from build123d import *

# Parameters (mm, degrees)
BOSS_EXTRUDE1_DEPTH      = 38
BOSS_EXTRUDE2_DEPTH      = 14
BOSS_EXTRUDE5_DEPTH      = 10
BOSS_EXTRUDE5_DEPTH_BACK = 38
SKETCH6_R                = 2
CUT_EXTRUDE2_DEPTH       = 36


with BuildPart() as part:
    # Sketch1 → Boss-Extrude1 (new body)
    with BuildSketch(Plane.XY):
        with BuildLine():
            Line((22.631743337, -14.12565234), (22.631743337, 13.87434766))
            Line((22.631743337, 13.87434766), (1.698298535, 18.39987252))
            ThreePointArc((1.698298535, 18.39987252), (-0.292783652, 18.720543399), (-2.306666921, 18.827838622))
            ThreePointArc((-2.306666921, 18.827838622), (-21.260157884, -0.12565234), (-2.306666921, -19.079143303))
            ThreePointArc((-2.306666921, -19.079143303), (-0.292783652, -18.971848079), (1.698298535, -18.651177201))
            Line((1.698298535, -18.651177201), (22.631743337, -14.12565234))
        make_face()
        with BuildLine():
            Line((17.644061285, -10.101016443), (17.644061285, 9.849711763))
            Line((17.644061285, 9.849711763), (0.644376893, 13.52481135))
            ThreePointArc((0.644376893, 13.52481135), (-0.822744568, 13.761096487), (-2.306666921, 13.840156571))
            ThreePointArc((-2.306666921, 13.840156571), (-16.272475832, -0.12565234), (-2.306666921, -14.091461251))
            ThreePointArc((-2.306666921, -14.091461251), (-0.822744568, -14.012401167), (0.644376893, -13.77611603))
            Line((0.644376893, -13.77611603), (17.644061285, -10.101016443))
        make_face(mode=Mode.SUBTRACT)
    extrude(amount=BOSS_EXTRUDE1_DEPTH)

    # Sketch2 → Boss-Extrude2 (add, symmetric)
    with BuildSketch(Plane(origin=(0, 0, 0), x_dir=(1, 0, 0), z_dir=(0, 1, 0))):
        Polygon((22.631743337, -38), (22.631743337, 0), (48.276983868, 0), (42.631743337, -38), align=None)
    extrude(amount=BOSS_EXTRUDE2_DEPTH, both=True)

    # Sketch4 → Boss-Extrude5 (add, two sides: drawn at the far end of the back side and taken through both)
    with BuildSketch(Plane(origin=(0, 14, 0), x_dir=(1, 0, 0), z_dir=(0, 1, 0)).offset(-BOSS_EXTRUDE5_DEPTH_BACK)):
        Polygon((28.899463429, 0), (22.957104975, -40), (48.666190602, -40), (54.608549056, 0), align=None)
    extrude(amount=BOSS_EXTRUDE5_DEPTH + BOSS_EXTRUDE5_DEPTH_BACK)

    # Sketch6 → Cut-Extrude2 (cut)
    with BuildSketch(Plane(origin=(28.275431305, 0, 4.200568706), x_dir=(-0.14694627579900546, 0, 0.9891444748007253), z_dir=(-0.9891444748007252, 0, -0.14694627579900543))):
        with Locations((0.974565013, 19)):
            Circle(SKETCH6_R)
        with Locations((29.583142195, 19)):
            Circle(SKETCH6_R)
        with Locations((0.974565013, -19)):
            Circle(SKETCH6_R)
        with Locations((29.583142195, -19)):
            Circle(SKETCH6_R)
    extrude(amount=-CUT_EXTRUDE2_DEPTH, mode=Mode.SUBTRACT)


solid = part.part
Read the model definition and answer for the solid it produces. Units are mm, in the model's axes. A direction names the side the tool comes from. Give positions to 0.01 mm unless a question says otherwise; leave off trailing zeros. Write each loop counter-clockwise with the first axis right and the second up, starting at its lowest first coordinate (ties: lowest second). Pieces come first, ordered by that corner, then holes. Notation, with made-up numbers: M 62,2.25 L 73,2.25 A31 cw 73,32.25 Z; hole C 88.5,88 d10. An arc over 180 degrees is marked long. One line per item, written item: value. Start each with the question number.
(1) Find the intervals of material crossed by line 1 (Z direction, x = -14, y = -15); line 2 (X direction, y = -2.5, z = 31.5); line 3 (Y direction, x = -5.5, z = 36), in increasing order.
(2) Find section C-C (z = 26.5). Determine the outline of the cut face in (x, y), plus the area to 3 significant figures.
(3) Find section D-D (y = -12). Determine the outline of the cut face in (x, z).
(4) Find section A-A (y = 16). Determine the outline of the cut face in (x, z).
(5) Determine the mould class of faces 1 (the cylindrical face through (36.367, 20.983, 35.047)), 2 (the flat face through (9.025, -11.964, 18.734)), 3 (the flat face through (25, 14, 15)), 4 (the flat face through (36, 0, 40)) for opening direction Y: pulls with the +Y half, pulls with the -Y half, needs draft (parallel to the pull), parting line crosses it, or undercut.
(6) A tool of negligible diameter and unlimited length cuts with its end or side. For faces 5 (the flat face through (25, -14, 15)), 6 (the flat face through (12.312, 16.105, 18.734)), 7 (the flat face through (12.02, -16.42, 18.73)), 8 (the flat face through (17.644, 0, 19)), from which of +Z, -Z, +X, -X, +Y, -Y can it reach the whole face along a straight path? Write none if from no direction.
(7) Flat-ended cylindrical pins translate along their axes: pin 1 Ø19 at (x, y) = (-4.5, 0.5) entering from +Z; pin 2 Ø4 at (x, y) = (6, 11) entering from +Z; pin 3 Ø3 at (y, z) = (-13.5, 16.5) entering from -X; pin 4 Ø1.5 at (y, z) = (14.5, 34) entering from +X. Find the tip coordinate at first contact, or state that the pin passes through.
(8) Find section B-B (x = -11.5). Determine the outline of the cut face in (y, z), plus the area to 3 significant figures.
Results below:
1. line 1: z = 0 to 38
1. line 2: x = -21.11 to -16.07, 17.64 to 49.93
1. line 3: y = -18.81 to -13.72, 13.47 to 18.56
2. outline: M 1.7,-18.65 L 22.63,-14.13 L 22.63,-14 L 24.96,-14 L 24.96,-24 L 50.67,-24 L 50.67,24 L 24.96,24 L 24.96,14 L 22.63,14 L 22.63,13.87 L 1.7,18.4 A18.95 ccw long Z; hole M 0.64,-13.78 L 17.64,-10.1 L 17.64,9.85 L 0.64,13.52 A13.97 ccw long Z
2. area: 1,910 mm^2
3. outline: M -17.08,0 L -9.66,0 L -9.66,38 L -17.08,38 Z; M 8.86,0 L 54.61,0 L 48.67,40 L 22.96,40 L 23.25,38 L 8.86,38 Z
4. outline: M -12.27,0 L 12.8,0 L 12.8,38 L -12.27,38 Z; M 22.96,40 L 28.9,0 L 54.61,0 L 48.67,40 Z
5. face 1: undercut
5. face 2: undercut
5. face 3: pulls with the +Y half
5. face 4: needs draft
6. face 5: -Z, -Y
6. face 6: +Z, -Z, +Y
6. face 7: +Z, -Z, -Y
6. face 8: +Z, -Z
7. pin 1: passes through
7. pin 2: stops at z = 38
7. pin 3: stops at x = -17.08
7. pin 4: stops at x = 49.67
8. outline: M -16.7,0 L -10.64,0 L -10.64,38 L -16.7,38 Z; M 10.39,0 L 16.45,0 L 16.45,38 L 10.39,38 Z
8. area: 461 mm^2
